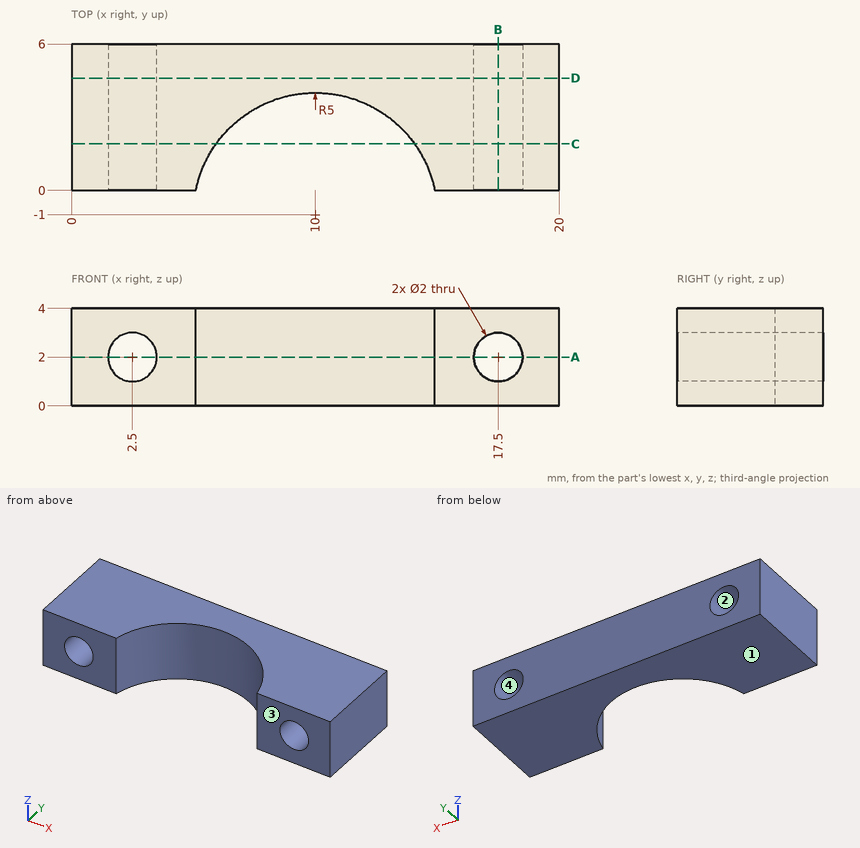
Answer from the drawing. Dimensions are ordinates in mm from the lowest x, y and z of the part. Coordinates: 2 decimals unless noted, no trailing zeros. Loops run counter-clockwise (first coordinate to the right, second up) from the corner with the lowest first, then second, coordinate; pieces in that order, holes last. Notation, with made-up numbers: (89.5, 14.25) - (115.5, 14.25) arc R31 ccw to (115.5, 50.25) - close; hole circle Ø10 at (-19.5, 71.25). An arc over 180 degrees is marked (long way). Use a Markdown table: item, result.
Item 1: Find section D-D, the plane y = 4.6. Determine the outline of the cut face in (x, z), and give its area (3 significant figures).
Evaluation:
| item | result |
|---|---|
| outline | (0, 0) - (20, 0) - (20, 4) - (0, 4) - close; hole circle Ø2 at (2.5, 2); hole circle Ø2 at (17.5, 2) |
| area | 73.7 mm2 |
Item 2: Find section C-C, the plane y = 1.9. Determine the outline of the cut face in (x, z), and give its area (3 significant figures).
Evaluation:
| item | result |
|---|---|
| outline | (0, 0) - (5.93, 0) - (5.93, 4) - (0, 4) - close; (14.07, 0) - (20, 0) - (20, 4) - (14.07, 4) - close; hole circle Ø2 at (2.5, 2); hole circle Ø2 at (17.5, 2) |
| area | 41.1 mm2 |
Item 3: The mould has two halves that part along Z. Classify the marked faces 1, 2, 3 and 4: +Z half, -Z half, draft (parallel to the pull), parting line (faces both ways), or undercut.
Evaluation:
| item | result |
|---|---|
| face 1 | -Z half |
| face 2 | undercut |
| face 3 | draft |
| face 4 | undercut |
Item 4: Find section A-A, the plane z = 2. Determine the outline of the cut face in (x, y), and give its area (3 significant figures).
Evaluation:
| item | result |
|---|---|
| outline | (0, 0) - (1.5, 0) - (1.5, 6) - (0, 6) - close; (3.5, 0) - (5.1, 0) arc R5 cw to (14.9, 0) - (16.5, 0) - (16.5, 6) - (3.5, 6) - close; (18.5, 0) - (20, 0) - (20, 6) - (18.5, 6) - close |
| area | 66.7 mm2 |
Item 5: Find section B-B, the plane x = 17.5. Determine the outline of the cut face in (y, z).
Evaluation:
| item | result |
|---|---|
| outline | (0, 0) - (6, 0) - (6, 1) - (0, 1) - close; (0, 3) - (6, 3) - (6, 4) - (0, 4) - close |
Item 6: Consider probe 1 along Z at (x, y) = (2.5, 2.5); probe 2 along X at (y, z) = (4.6, 1.6); probe 3 along X at (y, z) = (3.45, 1.6). Determine where each line is inside the solid, lowest interval first. Write a range as from..to.
Evaluation:
| item | result |
|---|---|
| probe 1 | z = 0..1, 3..4 |
| probe 2 | x = 0..1.58, 3.42..16.58, 18.42..20 |
| probe 3 | x = 0..1.58, 3.42..7.72, 12.28..16.58, 18.42..20 |
Item 7: Given pin 1 Ø1.8 at (x, z) = (2.5, 2) entering from -Y, flat-ended and moving along its own axis, determine where the tip first touches the part or whether it passes through.
Evaluation:
| item | result |
|---|---|
| pin 1 | passes through |
